from build123d import *

# Parameters (mm, degrees)
BOSS_EXTRUDE1_DEPTH = 503
CUT_EXTRUDE1_DEPTH  = 463
CUT_EXTRUDE2_DEPTH  = 28.6
LPATTERN1_COUNT     = 3
LPATTERN1_PITCH     = 177.2
LPATTERN1_COL_COUNT = 3
LPATTERN1_COL_PITCH = 177.2
SKETCH5_R           = 37.5
BOSS_EXTRUDE2_DEPTH = 50


with BuildPart() as part:
    # Sketch1 → Boss-Extrude1 (new, symmetric)
    with BuildSketch(Plane(origin=(0, 0, 0), x_dir=(0, 0, -1), z_dir=(1, 0, 0))):
        with BuildLine():
            Line((150, 0), (908, 0))
            Line((908, 0), (908, -25))
            Line((908, -25), (1068, -25))
            Line((1068, -25), (937.217045761, 22.601102492))
            Line((937.217045761, 22.601102492), (499.932588401, 780))
            Line((499.932588401, 780), (193.932588401, 780))
            Line((193.932588401, 780), (0, 300))
            Line((0, 300), (0, 150))
            ThreePointArc((0, 150), (43.933982822, 43.933982822), (150, 0))
        make_face()
    extrude(amount=BOSS_EXTRUDE1_DEPTH, both=True)

    # Sketch2 → Cut-Extrude1 (cut, symmetric)
    with BuildSketch(Plane(origin=(0, 0, 0), x_dir=(0, 0, -1), z_dir=(1, 0, 0))):
        with BuildLine():
            Line((908, 40), (1011.713283141, 40))
            Line((1011.713283141, 40), (1011.713283141, 740))
            Line((1011.713283141, 740), (499.932588401, 740))
            Line((499.932588401, 740), (220.912929075, 740))
            Line((220.912929075, 740), (40, 292.224787634))
            Line((40, 292.224787634), (40, 150))
            ThreePointArc((40, 150), (72.218254069, 72.218254069), (150, 40))
            Line((150, 40), (908, 40))
        make_face()
    extrude(amount=CUT_EXTRUDE1_DEPTH, both=True, mode=Mode.SUBTRACT)

    # Sketch3 → Cut-Extrude2 (cut, symmetric)
    with BuildSketch(Plane(origin=(0, 0, 0), x_dir=(0, 0, -1), z_dir=(1, 0, 0))):
        Polygon((946.796612299, 48.920745244), (905.079735991, -65.695430422), (1089.944771032, -65.695430422), (1089.944771032, 48.920745244), align=None)
    cut_extrude2 = extrude(amount=CUT_EXTRUDE2_DEPTH, both=True, mode=Mode.SUBTRACT)

    # LPattern1: Cut-Extrude2 ×3
    with Locations(*[(i * LPATTERN1_PITCH, 0, 0) for i in range(1, LPATTERN1_COUNT)]):
        add(cut_extrude2, mode=Mode.SUBTRACT)

    # LPattern1 col: Cut-Extrude2 ×3
    with Locations(*[(-i * LPATTERN1_COL_PITCH, 0, 0) for i in range(1, LPATTERN1_COL_COUNT)]):
        add(cut_extrude2, mode=Mode.SUBTRACT)

    # Sketch5 → Boss-Extrude2 (add)
    with BuildSketch(Plane(origin=(153, 0, 0), x_dir=(0, 0, -1), z_dir=(1, 0, 0))):
        with BuildLine():
            Line((49.932588401, 423.587493108), (49.932588401, 910))
            ThreePointArc((49.932588401, 910), (71.899579812, 963.033008589), (124.932588401, 985))
            Line((124.932588401, 985), (509.932588401, 985))
            ThreePointArc((509.932588401, 985), (574.884493685, 947.5), (574.884493685, 872.5))
            Line((574.884493685, 872.5), (510.706091093, 761.339745962))
            Line((510.706091093, 761.339745962), (499.932588401, 780))
            Line((499.932588401, 780), (193.932588401, 780))
            Line((193.932588401, 780), (49.932588401, 423.587493108))
        make_face()
        with Locations((124.932588401, 910)):
            Circle(SKETCH5_R, mode=Mode.SUBTRACT)
        with Locations((509.932588401, 910)):
            Circle(SKETCH5_R, mode=Mode.SUBTRACT)
    boss_extrude2 = extrude(amount=BOSS_EXTRUDE2_DEPTH)

    # Mirror1: Boss-Extrude2 across plane
    add(boss_extrude2.mirror(Plane(origin=(0, 0, 0), x_dir=(0, 0, 1), z_dir=(1, 0, 0))))


solid = part.part
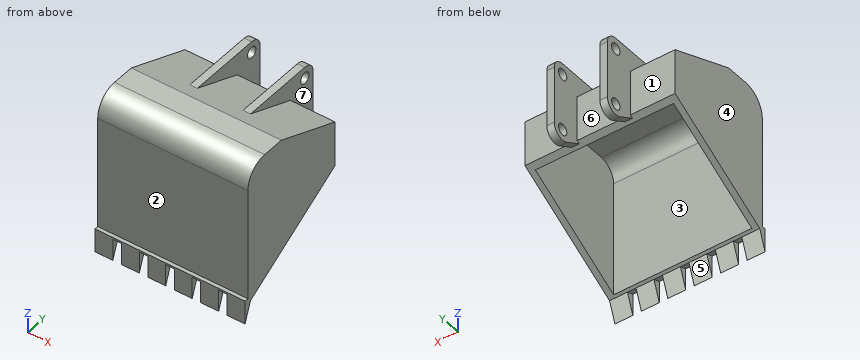
Read the model definition and answer for the solid it produces. Units are mm, in the model's axes. Face numbers are marked on the shaded views. A direction names the side the tool comes from. Give positions to 0.01 mm unless a question says otherwise; leave off trailing zeros. Write each loop counter-clockwise with the first axis right and the second up, starting at its lowest first coordinate (ties: lowest second). Pieces come first, ordered by that corner, then holes. Notation, with made-up numbers: (-23.5, 70.5) -> (9.5, 70.5) arc R21 cw to (9.5, 90.5) -> close; hole circle Ø8 at (27.5, 27.25). An arc over 180 degrees is marked (long way). Answer as a JSON object with one key per item and string values. Group by question number.
1) Each of these flat-tipped pins is pushed along its axis until it touches: P1, Ø14.5, axis at y = -2.5, z = -1025.5, coming from the -X side; P2, Ø10, axis at x = -248, y = 445.5, coming from the -Z side; P3, Ø8, axis at x = -39.5, y = 626, coming from the +Z side; P4, Ø1.5, axis at x = -185.5, z = -632, coming from the +Y side. Where does it stop, or does it pass through?
2) Find section D-D (y = 479). Write down the section's boundary in (x, z).
3) The mould has two halves that part along X. Classify the marked faces 5, 6 and 7: +X half, -X half, draft (parallel to the pull), parting line (faces both ways), or undercut.
4) A tool of negligible diameter and unlimited length cuts with its end or side. For the marked faces 1, 2, 3 and 4, from which of +Z, -Z, +X, -X, +Y, -Y can it reach the whole face along a straight path? Write none if from no direction.
5) Consider L1, parallel to Y at x = -78.5, z = -419.5; L2, parallel to X at y = 238, z = -385; L3, parallel to Y at x = 412, z = -564.5. Determine where each line is inside the solid, lowest interval first. Write a range as from..to.
6) Find section C-C (x = 69). Write down the section's boundary in (y, z).
7) Find section B-B (y = 847.5). Write down the section's boundary in (x, z), and give its area (3 significant figures).
8) Find section A-A (z = -341.5). Write down the section's boundary in (x, y), and give its area (3 significant figures).
Values follow:
{
 "1": {"P1": "stops at x = -503", "P2": "stops at z = -103.95", "P3": "stops at z = -130.1", "P4": "stops at y = 40"},
 "2": {"outline": "(-503, -673.72) -> (-463, -673.72) -> (-463, -115.46) -> (463, -115.46) -> (463, -673.72) -> (503, -673.72) -> (503, -72.32) -> (203, -72.32) -> (203, -49.93) -> (153, -49.93) -> (153, -72.32) -> (-153, -72.32) -> (-153, -49.93) -> (-203, -49.93) -> (-203, -72.32) -> (-503, -72.32) -> close"},
 "3": {"face 5": "draft", "face 6": "undercut", "face 7": "+X half"},
 "4": {"face 1": "+Z, -Z, -X, +Y", "face 2": "+Z, +X, -X, -Y", "face 3": "-Z", "face 4": "+Z, -Z, -X, +Y, -Y"},
 "5": {"L1": "y = 0..40, 740..780", "L2": "x = -503..-463, 463..503", "L3": "y = 0..40"},
 "6": {"outline": "(-25, -1068) -> (22.6, -937.22) -> (40, -927.17) -> (40, -150) arc R110 cw to (150, -40) -> (292.22, -40) -> (740, -220.91) -> (740, -523.03) -> (780, -499.93) -> (780, -193.93) -> (300, 0) -> (150, 0) arc R150 ccw to (0, -150) -> (0, -908) -> (-25, -908) -> close"},
 "7": {"outline": "(-203, -560.45) -> (-153, -560.45) -> (-153, -49.93) -> (-203, -49.93) -> close; (153, -560.45) -> (203, -560.45) -> (203, -49.93) -> (153, -49.93) -> close", "area": "51,100 mm2"},
 "8": {"outline": "(-503, 0) -> (503, 0) -> (503, 780) -> (203, 780) -> (203, 985) -> (153, 985) -> (153, 780) -> (-153, 780) -> (-153, 985) -> (-203, 985) -> (-203, 780) -> (-503, 780) -> close; hole (-463, 40) -> (463, 40) -> (463, 740) -> (-463, 740) -> close", "area": "157,000 mm2"}
}
